```python
from build123d import *

# Parameters (mm, degrees)
SKETCH2_R           = 7.5
BOSS_EXTRUDE3_DEPTH = 6
SKETCH4_R           = 30
BOSS_EXTRUDE6_DEPTH = 68
SKETCH5_R           = 15
CUT_EXTRUDE1_DEPTH  = 205.939015319
SKETCH6_R           = 21.472161424
CUT_EXTRUDE3_DEPTH  = 16
BOSS_EXTRUDE7_DEPTH = 45
FILLET2_R           = 15
SKETCH9_R           = 8
CUT_EXTRUDE8_DEPTH  = 17.5


with BuildPart() as part:
    # Sketch2 → Boss-Extrude3 (new, symmetric)
    with BuildSketch(Plane(origin=(0, 0, 0), x_dir=(1, 0, 0), z_dir=(0, 1, 0))):
        with BuildLine():
            Line((0, 15), (0, 85))
            ThreePointArc((0, 85), (4.393398282, 95.606601718), (15, 100))
            Line((15, 100), (66.502577388, 100))
            ThreePointArc((66.502577388, 100), (70.384863065, 99.488887394), (74.002577388, 97.990381057))
            Line((74.002577388, 97.990381057), (145, 57))
            ThreePointArc((145, 57), (160, 42), (145, 27))
            Line((145, 27), (122.393398282, 4.393398282))
            ThreePointArc((122.393398282, 4.393398282), (117.52704805, 1.141807012), (111.786796564, 0))
            Line((111.786796564, 0), (15, 0))
            ThreePointArc((15, 0), (4.393398282, 4.393398282), (0, 15))
        make_face()
        with Locations(Location((145, 42, 0), (0, 0, 270))):
            Circle(SKETCH2_R, mode=Mode.SUBTRACT)
        with Locations(Location((15, 85, 0), (0, 0, 270))):
            Circle(SKETCH2_R, mode=Mode.SUBTRACT)
        with Locations(Location((15, 15, 0), (0, 0, 270))):
            Circle(SKETCH2_R, mode=Mode.SUBTRACT)
    extrude(amount=BOSS_EXTRUDE3_DEPTH, both=True)

    # Sketch4 → Boss-Extrude6 (add)
    with BuildSketch(Plane(origin=(0, 6, 0), x_dir=(1, 0, 0), z_dir=(0, 1, 0))):
        with Locations(Location((50, 50, 0), (0, 0, 90))):
            Circle(SKETCH4_R)
    extrude(amount=BOSS_EXTRUDE6_DEPTH)

    # Sketch5 → Cut-Extrude1 (cut, through all)
    with BuildSketch(Plane(origin=(0, 74, 0), x_dir=(1, 0, 0), z_dir=(0, 1, 0))):
        with Locations(Location((49.557906347, 50.967812226, 0), (0, 0, 270))):
            Circle(SKETCH5_R)
    extrude(amount=-CUT_EXTRUDE1_DEPTH, mode=Mode.SUBTRACT)

    # Sketch6 → Cut-Extrude3 (cut)
    with BuildSketch(Plane(origin=(0, 74, 0), x_dir=(1, 0, 0), z_dir=(0, 1, 0))):
        with Locations(Location((49.557906347, 50.967812226, 0), (0, 0, 270))):
            Circle(SKETCH6_R)
    extrude(amount=-CUT_EXTRUDE3_DEPTH, mode=Mode.SUBTRACT)

    # Sketch8 → Boss-Extrude7 (add)
    with BuildSketch(Plane(origin=(0, 6, 0), x_dir=(1, 0, 0), z_dir=(0, 1, 0))):
        with BuildLine():
            Line((75.980762114, 65), (95, 65))
            Line((95, 65), (95, 50))
            Line((95, 50), (95, 35))
            Line((95, 35), (75.980762114, 35))
            ThreePointArc((75.980762114, 35), (20, 50), (75.980762114, 65))
        make_face()
    extrude(amount=BOSS_EXTRUDE7_DEPTH)

    # Fillet2
    # the kernel refuses this fillet: 15 mm, written as the material it takes off along each edge
    with BuildSketch(Plane(origin=(38.480762114, 51, -65), x_dir=(0, 0, 1), z_dir=(1, 0, 0))) as fillet2_piece_1_section:
        with BuildLine():
            CenterArc((FILLET2_R, FILLET2_R), FILLET2_R, 180, 90)
            Line((0, FILLET2_R), (0, 0))
            Line((0, 0), (FILLET2_R, 0))
        make_face()
    fillet2_piece_1 = extrude(amount=94.019237886, mode=Mode.PRIVATE)
    fillet2_piece_1 = fillet2_piece_1 - Plane(origin=(50, 47.545700525, -50), x_dir=(0, 0, -1), z_dir=(0, -1, 0)) * Cylinder(30, 249, mode=Mode.PRIVATE)
    add(fillet2_piece_1, mode=Mode.SUBTRACT)
    with BuildSketch(Plane(origin=(132.5, 51, -35), x_dir=(0, -1, 0), z_dir=(-1, 0, 0))) as fillet2_piece_2_section:
        with BuildLine():
            CenterArc((FILLET2_R, -FILLET2_R), FILLET2_R, 90, 90)
            Line((0, -FILLET2_R), (0, 0))
            Line((0, 0), (FILLET2_R, 0))
        make_face()
    fillet2_piece_2 = extrude(amount=94.019237886, mode=Mode.PRIVATE)
    fillet2_piece_2 = fillet2_piece_2 - Plane(origin=(50, 47.545704386, -50), x_dir=(0, 0, -1), z_dir=(0, -1, 0)) * Cylinder(30, 249, mode=Mode.PRIVATE)
    add(fillet2_piece_2, mode=Mode.SUBTRACT)

    # Sketch9 → Cut-Extrude8 (cut, symmetric)
    with BuildSketch(Plane(origin=(95, 0, 0), x_dir=(0, 0, -1), z_dir=(1, 0, 0))):
        with Locations((50, 36)):
            Circle(SKETCH9_R)
    extrude(amount=CUT_EXTRUDE8_DEPTH, both=True, mode=Mode.SUBTRACT)


solid = part.part
```
Geometry check sheet. Reference: the model listing, model coordinates, mm. A direction names the side the tool comes from. Give positions to 0.01 mm unless a question says otherwise; leave off trailing zeros. Order: outer loops, then holes, each group sorted by start corner. A loop starts at its lowest first (then second) coordinate and runs counter-clockwise, first axis right, second up. Notation, with made-up numbers: (53.5, 13.25) -> (102.5, 13.25) arc R17 ccw to (102.5, 28.25) -> close; hole circle Ø4 at (39, 14.25). An arc over 180 degrees is marked (long way). Write each question's results on one line, items separated by ' | '. Start each with the question number.
(1) Mould release check, pull along X, two halves, no side actions. Record for faces 6 (the face through (54.06, 0.08, -36.66)), 7 (the face through (81, 6, -28)), 8 (the face through (54.06, 54.55, -36.66)), 9 (the face through (95, 23, -50)): pulls with the +X half, pulls with the -X half, needs draft (parallel to the pull), parting line crosses it, or undercut.
(2) Gauge pin test, flat ends, axial feed: P1, Ø8, axis at y = 56, z = -13.5, coming from the +X side; P2, Ø18, axis at x = 49.56, z = -50.97, coming from the -Y side; P3, Ø3, axis at x = 81, y = 48, coming from the -Z side; P4, Ø13, axis at x = 54, z = -55.5, coming from the +Y side. Record the tip position at first contact, or that the pin passes through.
(3) Sectioned sample at C-C (y = 10.5). Enter the section's corners in (x, z).
(4) Sectioned sample at D-D (y = -1). Enter the section's corners in (x, z).
(5) Access from +Z, -Z, +X, -X, +Y, -Y to the whole of each face (thin tool, end or side, straight path). Record for faces 1 (the face through (50, 6, -51)), 2 (the face through (20.255, 39.524, -46.095)), 3 (the face through (77.5, 36, -50)), 4 (the face through (0, 0, -50)), 5 (the face through (87, 51, -50)).
(6) Scan lines: line 1 (X direction, y = 3, z = -42); line 2 (Y direction, x = 41, z = -93.5); line 3 (Z direction, x = 82.5, y = 7). Record each from-to range of solid material in increasing order.
(7) Sectioned sample at B-B (x = 150.5). Enter the section's corners in (y, z).
Answer below:
1) face 6: undercut | face 7: needs draft | face 8: undercut | face 9: pulls with the +X half
2) P1: through | P2: y = 6 | P3: z = -60.71 | P4: y = 51
3) outline: (75.98, -65) -> (95, -65) -> (95, -35) -> (75.98, -35) arc R30 ccw (long way) to start
4) outline: (0, -85) arc R15 ccw to (15, -100) -> (66.5, -100) arc R15 ccw to (74, -97.99) -> (145, -57) arc R15 ccw to (145, -27) -> (122.39, -4.39) arc R15 ccw to (111.79, 0) -> (15, 0) arc R15 ccw to (0, -15) -> close; hole circle Ø15 at (15, -85); hole circle Ø15 at (15, -15); hole circle Ø30 at (49.56, -50.97); hole circle Ø15 at (145, -42)
5) face 1: -Y | face 2: +Y | face 3: +X | face 4: +Z, -Z, -X, +Y, -Y | face 5: +X, +Y
6) line 1: 0 to 37.53, 61.58 to 137.5, 152.5 to 160 | line 2: -6 to 6 | line 3: -65 to -35
7) outline: (-6, -55.96) -> (6, -55.96) -> (6, -47.1) -> (-6, -47.1) -> close; (-6, -36.9) -> (6, -36.9) -> (6, -28.04) -> (-6, -28.04) -> close
